The drawing under review shows one solid part. Ordinate dimensions are in mm from its lowest x, y, z. A direction names the side the tool comes from. Coordinates: 2 decimals unless noted, no trailing zeros. Write each loop counter-clockwise with the first axis right and the second up, starting at its lowest first coordinate (ties: lowest second). Pieces come first, ordered by that corner, then holes.
Q1. Insertion check: pin 1 (3.5 mm diameter, centred on x = 55.75, y = 4.25, fed in from +Z); pin 2 (10 mm diameter, centred on x = 51.5, y = 51.5, fed in from -Z); pin 3 (3 mm diameter, centred on x = 21, y = 37, fed in from +Z). Each pin has a flat end and moves straight along its axis. Give the tip position at first contact, or say it passes through.
Q2. Take a section at D-D (y = 4.25). Give the boundary of the cut face in (x, z), and give its area (3 significant figures).
Q3. Take a section at C-C (x = 4.25). Give the boundary of the cut face in (y, z).
Q4. Take a section at A-A (x = 15). Give the boundary of the cut face in (y, z), and give its area (3 significant figures).
Q5. For probe 1 along Y at (x, z) = (4.25, 18.55); probe 2 along Y at (x, z) = (50, 16.75), list the stretches that pass through material, from the lowest coordinate up.
Q6. Machinability: for the marked faces 4, 5 and 6, which of the approach directions +Z, -Z, +X, -X, +Y, -Y give a long, thin tool a straight path to every point of the face, cutting with its end or side? Answer none if there is none.
Q7. Mouldability with a two-part tool opening along Y and no side actions: class the marked faces 1, 2 and 3 as pulls with the +Y half, pulls with the -Y half, needs draft (parallel to the pull), parting line crosses it, or undercut.
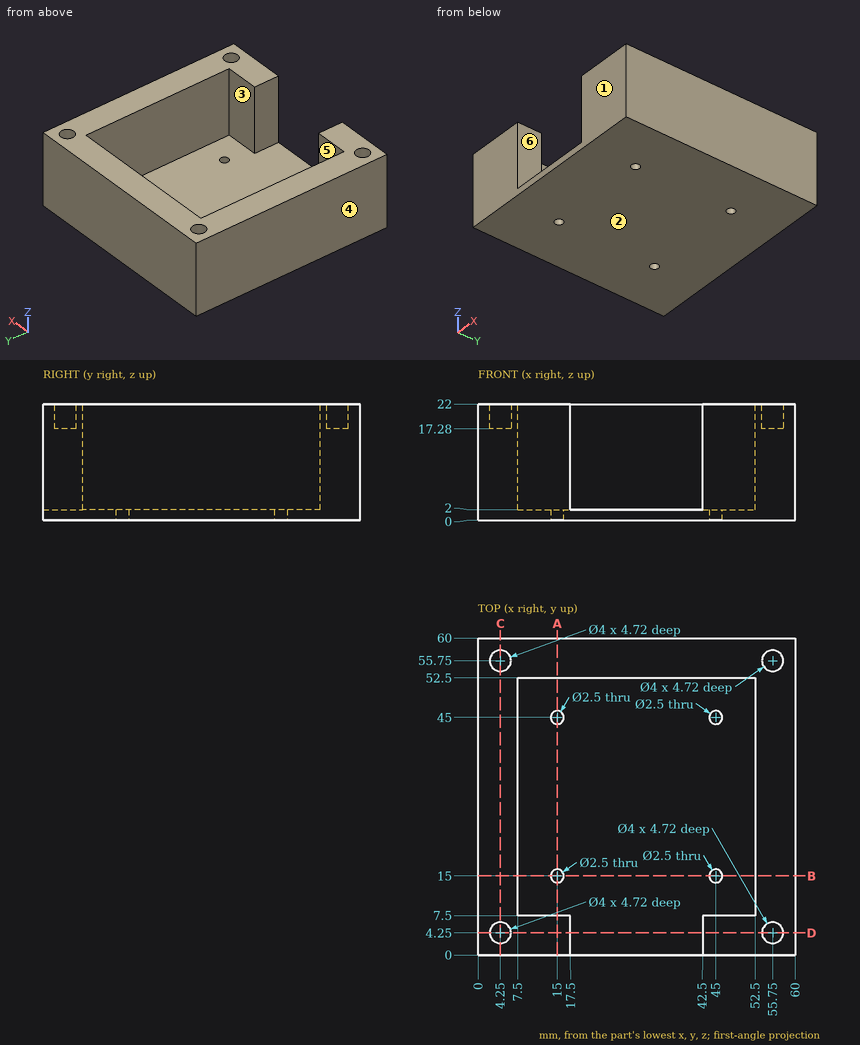
Response:
1. pin 1: stops at z = 17.28
1. pin 2: stops at z = 0
1. pin 3: stops at z = 2
2. outline: (0, 0) - (60, 0) - (60, 22) - (57.75, 22) - (57.75, 17.28) - (53.75, 17.28) - (53.75, 22) - (42.5, 22) - (42.5, 2) - (17.5, 2) - (17.5, 22) - (6.25, 22) - (6.25, 17.28) - (2.25, 17.28) - (2.25, 22) - (0, 22) - close
2. area: 782 mm2
3. outline: (0, 0) - (60, 0) - (60, 22) - (57.75, 22) - (57.75, 17.28) - (53.75, 17.28) - (53.75, 22) - (6.25, 22) - (6.25, 17.28) - (2.25, 17.28) - (2.25, 22) - (0, 22) - close
4. outline: (0, 0) - (13.75, 0) - (13.75, 2) - (7.5, 2) - (7.5, 22) - (0, 22) - close; (16.25, 0) - (43.75, 0) - (43.75, 2) - (16.25, 2) - close; (46.25, 0) - (60, 0) - (60, 22) - (52.5, 22) - (52.5, 2) - (46.25, 2) - close
4. area: 410 mm2
5. probe 1: y = 0 to 2.25, 6.25 to 53.75, 57.75 to 60
5. probe 2: y = 0 to 7.5, 52.5 to 60
6. face 4: +Z, -Z, -X, +Y, -Y
6. face 5: +Z
6. face 6: +Z, -Y
7. face 1: pulls with the -Y half
7. face 2: needs draft
7. face 3: undercut
